Could you check a few things on this model? Use its own coordinates, in mm. Give positions to 0.01 mm unless a question says otherwise; leave off trailing zeros. Write each loop counter-clockwise with the first axis right and the second up, starting at its lowest first coordinate (ties: lowest second). Pieces come first, ordered by that corner, then holes. Notation, with made-up numbers: (-1, 12.25) - (18, 12.25) arc R22 cw to (18, 44.25) - close; hole circle Ø8 at (87.5, 5.5). An arc over 180 degrees is marked (long way). Use one line per item in the form item = value.
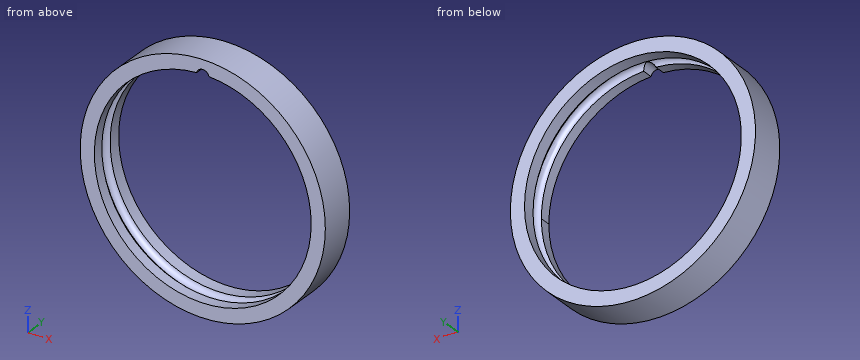
```python
from build123d import *

# Parameters (mm, degrees)
CYLINDER2620_R     = 2
CYLINDER2620_DEPTH = 10
TORUS004_R         = 2
TUBE115_R          = 39
TUBE115_R_2        = 34.5
TUBE115_DEPTH      = 11.5


with BuildPart() as obj1:
    # Cylinder2620 → Cylinder2620 (new body)
    with BuildSketch(Plane(origin=(17, -98, 44), x_dir=(1, 0, 0), z_dir=(0, -1, 0))):
        Circle(CYLINDER2620_R)
    extrude(amount=CYLINDER2620_DEPTH)


with BuildPart() as obj2:
    # Torus004 → Torus004 (revolve)
    with BuildSketch(Plane(origin=(17, -98, 10), x_dir=(1, 0, 0), z_dir=(0, 0, -1))):
        with Locations((34.1, 0)):
            Circle(TORUS004_R)
    revolve(axis=Axis((17, -98, 10), (0, -1, 0)))


with BuildPart() as cut970:
    # Tube115 → Tube115 (new body)
    with BuildSketch(Plane(origin=(17, -92, 10), x_dir=(1, 0, 0), z_dir=(0, -1, 0))):
        Circle(TUBE115_R)
        Circle(TUBE115_R_2, mode=Mode.SUBTRACT)
    extrude(amount=TUBE115_DEPTH)

    # Cut969: cut obj2
    add(obj2.part, mode=Mode.SUBTRACT)

    # Cut970: cut obj1
    add(obj1.part, mode=Mode.SUBTRACT)


with BuildPart() as cut970_1:
    # Cut970 placement: moved
    add(cut970.part.moved(Location((0, -2, 0))))


solid = cut970_1.part
```
1. Imagine slicing it at B-B, the plane y = -103.5. List the corners of the cut face in (x, z) for me.
Response values:
outline = circle Ø78 at (17, 10); hole (15.05, 44.44) arc R34.5 ccw (long way) to (18.95, 44.44) arc R2 ccw to start
2. If I drill on line 1 (Z direction, x = 17, y = -104.25); line 2 (Z direction, x = 17, y = -95); line 3 (X direction, y = -94.5, z = 36), over which ranges is the centre line in solid material (lowest first)? Write a range as from..to.
Response values:
line_1 = -29..-24.5, 46..49
line_2 = -29..-24.5, 44.5..49
line_3 = -12.07..-5.68, 39.68..46.07
3. For pin 1 (3 mm diameter, centred on y = -98.5, z = -4, fed in from +X); pin 2 (1 mm diameter, centred on x = 20, y = -96.5, fed in from +Z); pin 3 (1.5 mm diameter, centred on x = 7, y = -98, fed in from +Z), each with a flat end and sliding along its axis, tell me the tip position at first contact or that it passes through.
Response values:
pin_1 = 53.94
pin_2 = 48.92
pin_3 = 47.89
4. Imagine slicing it at A-A, the plane x = 17. List the corners of the cut face in (y, z) for me.
Response values:
outline = (-105.5, -29) - (-94, -29) - (-94, -24.5) - (-98.04, -24.5) arc R2 cw to (-101.96, -24.5) - (-105.5, -24.5) - close; (-105.5, 46) - (-100.62, 46) arc R2 cw to (-98.04, 44.5) - (-94, 44.5) - (-94, 49) - (-105.5, 49) - close
